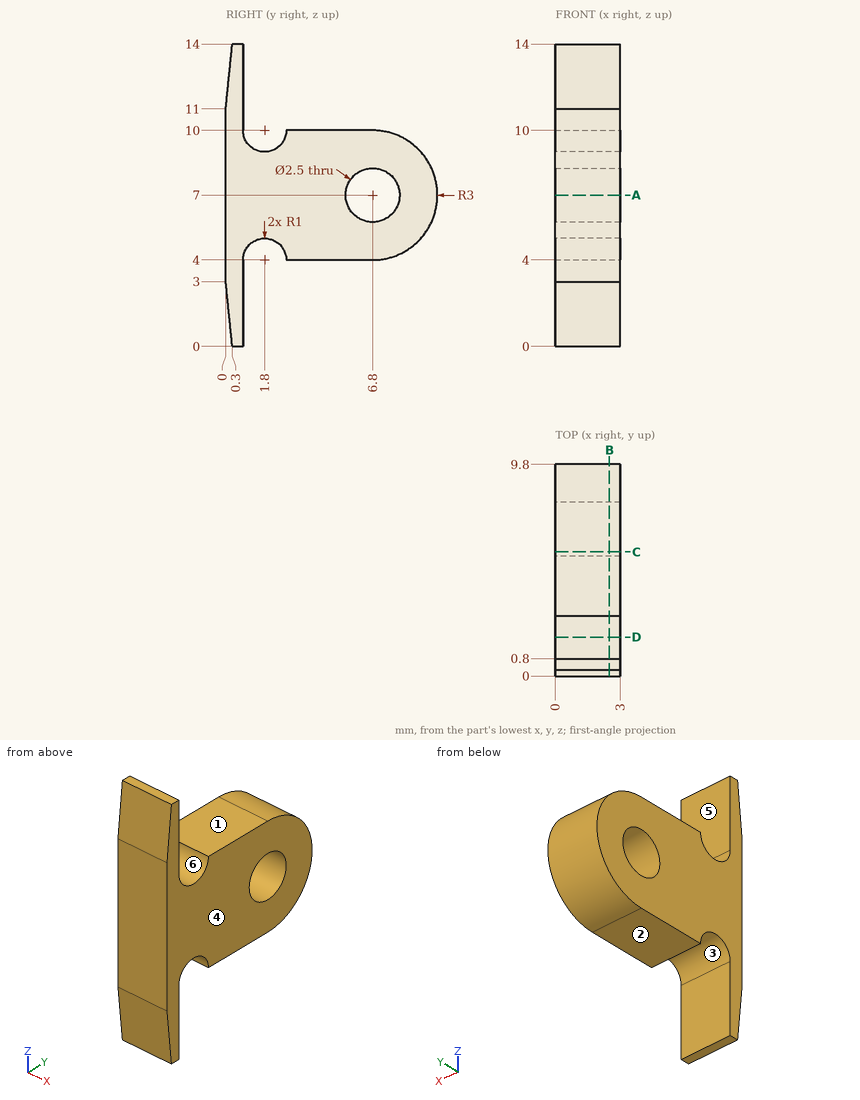
Answer from the drawing. Dimensions are ordinates in mm from the lowest x, y and z of the part. A direction names the side the tool comes from. Coordinates: 2 decimals unless noted, no trailing zeros. Loops run counter-clockwise (first coordinate to the right, second up) from the corner with the lowest first, then second, coordinate; pieces in that order, holes last. Notation, with made-up numbers: (-26, 30) - (32, 30) arc R26 cw to (32, 62) - close; hole circle Ø8 at (-37, 15). An arc over 180 degrees is marked (long way). Use a Markdown table: item, result.
Item 1: The mould has two halves that part along Y. Classify the marked faces 4, 5 and 6: +Y half, -Y half, draft (parallel to the pull), parting line (faces both ways), or undercut.
Evaluation:
| item | result |
|---|---|
| face 4 | draft |
| face 5 | +Y half |
| face 6 | undercut |
Item 2: Find section C-C, the plane y = 5.75. Determine the outline of the cut face in (x, z).
Evaluation:
| item | result |
|---|---|
| outline | (0, 4) - (3, 4) - (3, 6.32) - (0, 6.32) - close; (0, 7.68) - (3, 7.68) - (3, 10) - (0, 10) - close |
Item 3: Find section B-B, the plane x = 2.5. Determine the outline of the cut face in (y, z).
Evaluation:
| item | result |
|---|---|
| outline | (0, 3) - (0.3, 0) - (0.8, 0) - (0.8, 4) arc R1 cw to (2.8, 4) - (6.8, 4) arc R3 ccw to (6.8, 10) - (2.8, 10) arc R1 cw to (0.8, 10) - (0.8, 14) - (0.3, 14) - (0, 11) - close; hole circle Ø2.5 at (6.8, 7) |
Item 4: Find section A-A, the plane z = 7. Determine the outline of the cut face in (x, y), and give its area (3 significant figures).
Evaluation:
| item | result |
|---|---|
| outline | (0, 0) - (3, 0) - (3, 5.55) - (0, 5.55) - close; (0, 8.05) - (3, 8.05) - (3, 9.8) - (0, 9.8) - close |
| area | 21.9 mm2 |
Item 5: Consider probe 1 along Y at (x, z) = (2.3, 7); probe 2 along Y at (x, z) = (2.2, 6.25); probe 3 along Z at (x, y) = (2.25, 6.5). Determine where each line is inside the solid, lowest interval first. Write a range as from..to.
Evaluation:
| item | result |
|---|---|
| probe 1 | y = 0..5.55, 8.05..9.8 |
| probe 2 | y = 0..5.8, 7.8..9.7 |
| probe 3 | z = 4..5.79, 8.21..10 |
Item 6: Find section D-D, the plane y = 1.8. Determine the outline of the cut face in (x, z), and give its area (3 significant figures).
Evaluation:
| item | result |
|---|---|
| outline | (0, 5) - (3, 5) - (3, 9) - (0, 9) - close |
| area | 12.0 mm2 |
Item 7: Given pin 1 Ø1 at (x, y) = (1.5, 8) entering from +Z; pin 2 Ø0.9 at (x, y) = (1, 4) entering from +Z; pin 3 Ø1.5 at (x, z) = (1.5, 12) entering from +Y, each flat-ended and moving along its own axis, determine where each tip first touches the part or whether it passes through.
Evaluation:
| item | result |
|---|---|
| pin 1 | stops at z = 9.92 |
| pin 2 | stops at z = 10 |
| pin 3 | stops at y = 0.8 |
Item 8: For the marked faces 1, 2 and 3, determine the directions among +Z, -Z, +X, -X, +Y, -Y from which every point of the face is accessible in a straight line to the end or side of a thin tool.
Evaluation:
| item | result |
|---|---|
| face 1 | +Z, +X, -X, +Y |
| face 2 | -Z, +X, -X, +Y |
| face 3 | -Z, +X, -X |
